Part model, mm, in its own coordinate system. Face numbers are marked on the shaded views. A direction names the side the tool comes from. Give positions to 0.01 mm unless a question says otherwise; leave off trailing zeros. Loops run counter-clockwise (first coordinate to the right, second up) from the corner with the lowest first, then second, coordinate; pieces in that order, holes last. Notation, with made-up numbers: (43.25, 79) -> (71.25, 79) arc R22 ccw to (71.25, 104) -> close; hole circle Ø3 at (-0.75, 61). An arc over 180 degrees is marked (long way). Write item = value, one per line.
from build123d import *

# Parameters (mm, degrees)
SKETCH1_R           = 3.96875
BOSS_EXTRUDE1_DEPTH = 30.1625


with BuildPart() as part:
    # Sketch1 → Boss-Extrude1 (new body)
    with BuildSketch(Plane.XY):
        Polygon((3.175, 13.49375), (-3.175, 13.49375), (-7.9375, 8.73125), (-16.66875, 8.73125), (-16.66875, -8.73125), (16.66875, -8.73125), (16.66875, 8.73125), (7.9375, 8.73125), align=None)
        with Locations(Location((0, 0, 0), (0, 0, 180))):
            Circle(SKETCH1_R, mode=Mode.SUBTRACT)
    extrude(amount=BOSS_EXTRUDE1_DEPTH)


solid = part.part
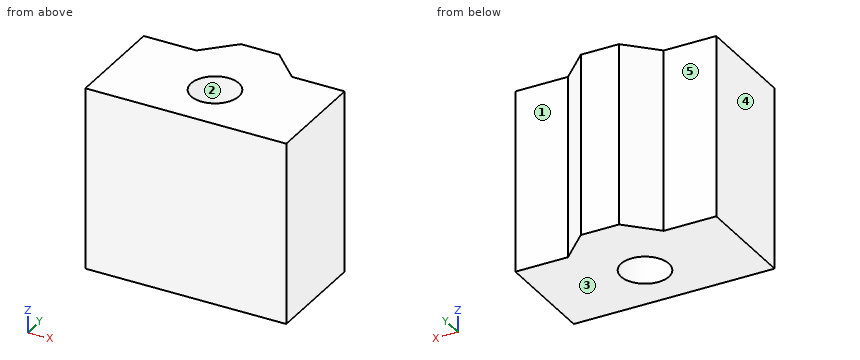
1) Slice it at B-B, the plane z = 21.5. List the corners of the cut face in (x, y) (1 decimal).
Resolved:
outline = (-16.7, -8.7) -> (16.7, -8.7) -> (16.7, 8.7) -> (7.9, 8.7) -> (3.2, 13.5) -> (-3.2, 13.5) -> (-7.9, 8.7) -> (-16.7, 8.7) -> close; hole circle Ø7.9 at (0, 0)
2) Drop flat-ended pins along their axis: P1, Ø2.5, axis at x = -10.5, z = 16.5, coming from the +Y side; P2, Ø10, axis at x = -10.5, z = 20.5, coming from the +Y side. Give the stop position or say it passes through.
Resolved:
P1 = 8.73
P2 = 11.17
3) Which spindle directions (+Z, -Z, +X, -X, +Y, -Y) get a long thin tool onto all of the face, cutting with end or side? Do the marked faces 4 and 5. Say none if no direction does.
Resolved:
face_4 = +Z, -Z, -X, +Y, -Y
face_5 = +Z, -Z, -X, +Y
4) Slice it at D-D, the plane x = -12. List the corners of the cut face in (y, z), and give its area (3 significant figures).
Resolved:
outline = (-8.73, 0) -> (8.73, 0) -> (8.73, 30.16) -> (-8.73, 30.16) -> close
area = 527 mm²
5) Slice it at A-A, the plane x = 0. List the corners of the cut face in (y, z).
Resolved:
outline = (-8.73, 0) -> (-3.97, 0) -> (-3.97, 30.16) -> (-8.73, 30.16) -> close; (3.97, 0) -> (13.49, 0) -> (13.49, 30.16) -> (3.97, 30.16) -> close
6) Pull direction Y, two halves, no side cores. Call the marked faces 1, 2 and 3: pulls with the +Y half, pulls with the -Y half, needs draft (parallel to the pull), parting line crosses it, or undercut.
Resolved:
face_1 = pulls with the +Y half
face_2 = undercut
face_3 = needs draft
7) Slice it at C-C, the plane y = 0. List the corners of the cut face in (x, z).
Resolved:
outline = (-16.67, 0) -> (-3.97, 0) -> (-3.97, 30.16) -> (-16.67, 30.16) -> close; (3.97, 0) -> (16.67, 0) -> (16.67, 30.16) -> (3.97, 30.16) -> close
8) Drill centre lines: line 1 along Y through (x, z) = (0, 23); line 2 along X through (y, z) = (-0.25, 5.5); line 3 along X through (y, z) = (-1.5, 20). Where is each one in solid material? Low to high. Write a range as [from, to].
Resolved:
line_1 = [-8.73, -3.97], [3.97, 13.49]
line_2 = [-16.67, -3.96], [3.96, 16.67]
line_3 = [-16.67, -3.67], [3.67, 16.67]
